Autodesk Inventor part; units mm, degrees
ref_plane "YZ Plane" through (0, 0, 0) normal (1, 0, 0) x (0, 1, 0)
ref_plane "XZ Plane" through (0, 0, 0) normal (0, 1, 0) x (-1, 0, 0)
ref_plane "XY Plane" through (0, 0, 0) normal (0, 0, 1) x (1, 0, 0)
sketch "Sketch1" plane through (0, 0, 0) normal (1, 0, 0) x (0, 1, 0)
  line L0 (-8.0203, -13.1567) -> (-48.0203, -13.1567)
  line L1 (-48.0203, -13.1567) -> (-48.0203, -19.1567)
  line L2 (-48.0203, -19.1567) -> (-8.0203, -19.1567)
  line L3 (-3.0203, -24.1567) -> (-3.0203, -144.1567)
  line L4 (-3.0203, -144.1567) -> (6.9797, -144.1567)
  line L5 (6.9797, -144.1567) -> (6.9797, -24.1567)
  arc A0 (6.9797, -24.1567) -> (-8.0203, -13.1567) centre (-7.4798, -28.147) ccw
  arc A1 (-3.0203, -24.1567) -> (-8.0203, -19.1567) centre (-8.0203, -24.1567) ccw
  point P0 (0, 0)
  dimension "d2" = 40
  dimension "d5" = 6
  dimension "d15" = 120
  dimension "d16" = 10
  dimension "d19" = 15
  dimension "d20" = 5
extrude "Extrusion1" add sketch "Sketch1" along normal blind 150
sketch "Sketch2" plane through (0, -48.0203, -13.1567) normal (0, 0, 1) x (1, 0, 0)
  line L0 (30, 38) -> (120, 38)
  line L1 (120, 38) -> (120, -15.5969)
  line L2 (120, -15.5969) -> (30, -15.5969)
  line L3 (30, -15.5969) -> (30, 38)
  line L4 (0, 40) -> (150, 40)
  line L5 (0, 40) -> (0, 0)
  point P0 (0, 48.0203)
  dimension "d10" = 2
  dimension "d11" = 30
  dimension "d12" = 90
extrude "Extrusion2" cut sketch "Sketch2" against normal blind 150
sketch "Sketch3" plane through (150, 0, 0) normal (1, 0, 0) x (0, 0, -1)
  line L0 (144.1567, 6.9797) -> (24.1567, 6.9797)
  point P0 (0, 0)
sketch "Sketch4" plane through (0, 6.9797, -24.1567) normal (0, 1, 0) x (1, 0, 0)
  line L0 (150, 120) -> (150, 0)
  line L1 (150, 120) -> (80, 120)
  line L2 (80, 120) -> (80, 50)
  line L3 (80, 50) -> (150, 50)
  line L4 (150, 50) -> (150, 120)
  point P0 (0, -24.1567)
  dimension "d31" = 70
  dimension "d32" = 70
extrude "Extrusion3" add sketch "Sketch4" along normal blind 200
sketch "Sketch5" plane through (0, 206.9797, -24.1567) normal (0, 1, 0) x (1, 0, 0)
  line L0 (84, 54) -> (146, 54)
  line L1 (146, 54) -> (146, 116)
  line L2 (146, 116) -> (84, 116)
  line L3 (84, 116) -> (84, 54)
  line L4 (150, 120) -> (80, 120)
  line L5 (150, 50) -> (150, 120)
  point P0 (0, -24.1567)
  dimension "d35" = 62
  dimension "d36" = 62
  dimension "d37" = 4
  dimension "d38" = 4
extrude "Extrusion4" cut sketch "Sketch5" against normal blind 150
sketch "Sketch6" plane through (150, 0, 0) normal (1, 0, 0) x (0, 0, -1)
  line L0 (78.1567, 6.9797) -> (140.1567, 6.9797)
  line L1 (140.1567, 6.9797) -> (140.1567, 56.9797)
  line L2 (140.1567, 56.9797) -> (78.1567, 56.9797)
  line L3 (78.1567, 56.9797) -> (78.1567, 6.9797)
  line L4 (144.1567, -3.0203) -> (144.1567, 206.9797)
  line L5 (74.1567, 6.9797) -> (144.1567, 6.9797)
  point P0 (0, 0)
  dimension "d41" = 50
  dimension "d42" = 62
  dimension "d43" = 4
  dimension "d47" = 0
extrude "Extrusion5" cut sketch "Sketch6" against normal blind 150
sketch "Sketch8" plane through (80, 6.9797, -74.1567) normal (0, 0, 1) x (1, 0, 0)
  line L0 (15, 34.7846) -> (20, 34.7846)
  line L1 (20, 34.7846) -> (20, 4.7846)
  line L2 (20, 4.7846) -> (15, 4.7846)
  line L3 (15, 4.7846) -> (15, 34.7846)
  line L4 (30, 34.7846) -> (35, 34.7846)
  line L5 (35, 34.7846) -> (35, 4.7846)
  line L6 (35, 4.7846) -> (30, 4.7846)
  line L7 (30, 4.7846) -> (30, 34.7846)
  line L8 (45, 34.7846) -> (50, 34.7846)
  line L9 (50, 34.7846) -> (50, 4.7846)
  line L10 (50, 4.7846) -> (45, 4.7846)
  line L11 (45, 4.7846) -> (45, 34.7846)
  line L12 (0, 0) -> (0, 200)
  point P0 (-80, -6.9797)
  dimension "d48" = 5
  dimension "d49" = 30
  dimension "d50" = 5
  dimension "d51" = 30
  dimension "d52" = 5
  dimension "d53" = 30
  dimension "d54" = 0
  dimension "d55" = 0
  dimension "d56" = 10
  dimension "d57" = 10
  dimension "d58" = 15
extrude "Extrusion6" cut sketch "Sketch8" against normal through all
sketch "Sketch9" plane through (80, 6.9797, -74.1567) normal (0, 0, 1) x (1, 0, 0)
  line L0 (0, 180) -> (15, 180)
  line L1 (15, 180) -> (15, 70)
  line L2 (15, 70) -> (0, 70)
  line L3 (0, 70) -> (0, 180)
  line L4 (0, 0) -> (0, 200)
  line L5 (55, 180) -> (70, 180)
  line L6 (70, 180) -> (70, 70)
  line L7 (70, 70) -> (55, 70)
  line L8 (55, 70) -> (55, 180)
  line L9 (70, 0) -> (70, 200)
  line L10 (0, 200) -> (70, 200)
  point P0 (-80, -6.9797)
  dimension "d61" = 0
  dimension "d62" = 15
  dimension "d63" = 110
  dimension "d64" = 15
  dimension "d65" = 110
  dimension "d66" = 0
  dimension "d67" = 0
  dimension "d80" = 20
extrude "Extrusion7" cut sketch "Sketch9" against normal blind 15
sketch "Sketch11" plane through (0, -3.0203, -144.1567) normal (0, 0, -1) x (-1, 0, 0)
  line L0 (-80, 10) -> (-80, 210)
  line L1 (-80, 190) -> (-95, 190)
  line L2 (-95, 190) -> (-95, 80)
  line L3 (-95, 80) -> (-80, 80)
  line L4 (-80, 80) -> (-80, 190)
  line L5 (-135, 190) -> (-150, 190)
  line L6 (-150, 190) -> (-150, 80)
  line L7 (-150, 80) -> (-135, 80)
  line L8 (-135, 80) -> (-135, 190)
  line L9 (-150, 0) -> (-150, 210)
  point P0 (0, 3.0203)
  point P1 (-80, 190)
  point P2 (-110.828, 190)
  point P3 (-80, 80)
  dimension "d71" = 110
  dimension "d72" = 0
  dimension "d73" = 15
  dimension "d74" = 110
  dimension "d75" = 0
  dimension "d76" = 15
  dimension "d77" = 0
  dimension "d81" = 0
extrude "Extrusion8" cut sketch "Sketch11" against normal blind 15
properties part number "Housing"
Input: part model. Units: mm. Frame: model coordinates. A direction names the side the tool comes from. Coordinates: 2 decimals unless noted, no trailing zeros. Order: outer loops, then holes, each group sorted by start corner. A loop starts at its lowest first (then second) coordinate and runs counter-clockwise, first axis right, second up. Notation, with made-up numbers: M -25,31 L -9,31 A25 ccw -9,44 Z; hole C 13.25,18.5 d7. An arc over 180 degrees is marked long. Answer in a Markdown table with one row per item.
(1) Draft query along Y for faces 1 (the flat face through (80, 128, -110)), 2 (the flat face through (83.7, 206.98, -114.5)), 3 (the cylindrical face through (73.95, -4.524, -20.583)), 4 (the flat face through (84, 76.98, -142)). Return one class per face: pulls with the +Y half, pulls with the -Y half, needs draft (parallel to the pull), parting line crosses it, or undercut.
Numbers:
| item | result |
|---|---|
| face 1 | needs draft |
| face 2 | pulls with the +Y half |
| face 3 | pulls with the -Y half |
| face 4 | undercut |
(2) Material intervals for line 1 (X direction, y = 143.5, z = -95); line 2 (Z direction, x = 106, y = 74); line 3 (Y direction, x = 7, z = -104.5), sorted ascending. Write a range as [from, to].
Numbers:
| item | result |
|---|---|
| line 1 | x = [80, 84], [146, 150] |
| line 2 | z = [-144.16, -140.16], [-78.16, -74.16] |
| line 3 | y = [-3.02, 6.98] |
(3) Section query D-D, the plane y = 21.5. Give the number of separate pieces and of enclosed holes in the cut face, plus the area to 3 significant figures.
Numbers:
| item | result |
|---|---|
| separate pieces | 8 |
| enclosed holes | 0 |
| area | 440 mm^2 |
(4) Contact query for flat-ended pins moving along their axis: pin 1 Ø3 at (y, z) = (147.5, -75.5) entering from +X; pin 2 Ø2 at (x, y) = (90, 36.5) entering from +Z; pin 3 Ø1.5 at (x, z) = (21, -55) entering from -Y. Output: stop coordinate, or through.
Numbers:
| item | result |
|---|---|
| pin 1 | stops at x = 135 |
| pin 2 | stops at z = -74.16 |
| pin 3 | stops at y = -3.02 |
(5) Section query C-C, the plane y = 177. Output: boundary loops of the cut face in (x, z).
Numbers:
| item | result |
|---|---|
| outline | M 80,-129.16 L 84,-129.16 L 84,-89.16 L 80,-89.16 Z; M 95,-144.16 L 135,-144.16 L 135,-140.16 L 95,-140.16 Z; M 95,-78.16 L 135,-78.16 L 135,-74.16 L 95,-74.16 Z; M 146,-129.16 L 150,-129.16 L 150,-89.16 L 146,-89.16 Z |
(6) Section query A-A, the plane x = 89. Output: boundary loops of the cut face in (y, z).
Numbers:
| item | result |
|---|---|
| outline | M -10.02,-19.16 L -8.02,-19.16 A5 cw -3.02,-24.16 L -3.02,-144.16 L 76.98,-144.16 L 76.98,-140.16 L 6.98,-140.16 L 6.98,-78.16 L 76.98,-78.16 L 76.98,-74.16 L 6.98,-74.16 L 6.98,-24.16 A15 ccw -8.02,-13.16 L -10.02,-13.16 Z; M 186.98,-144.16 L 206.98,-144.16 L 206.98,-140.16 L 186.98,-140.16 Z; M 186.98,-78.16 L 206.98,-78.16 L 206.98,-74.16 L 186.98,-74.16 Z |
(7) Section query B-B, the plane z = -104. Output: boundary loops of the cut face in (x, y), plus the area to 3 significant figures.
Numbers:
| item | result |
|---|---|
| outline | M 0,-3.02 L 150,-3.02 L 150,6.98 L 0,6.98 Z; M 80,56.98 L 84,56.98 L 84,206.98 L 80,206.98 Z; M 146,56.98 L 150,56.98 L 150,206.98 L 146,206.98 Z |
| area | 2,700 mm^2 |
(8) Access query for faces 5 (the flat face through (115, 106, -74.157)), 6 (the flat face through (24, -28, -19.157)), 7 (the flat face through (84, 76.98, -77)), 8 (the flat face through (146, 133, -109)). Directions: +Z, -Z, +X, -X, +Y, -Y. A direction counts if a zero-diameter tool reaches every point of the face in a straight line with its end or side. Return the directions, or none.
Numbers:
| item | result |
|---|---|
| face 5 | +Z, +X, -X, +Y |
| face 6 | -Z, +X, -X, -Y |
| face 7 | +Z, -X |
| face 8 | +Y |
